Input: dimensioned drawing with shaded views. Units: mm. Origin: part minimum x, y, z. A direction names the side the tool comes from. Round coordinates to 2 decimals unless told otherwise and drop trailing zeros. Order: outer loops, then holes, each group sorted by start corner. A loop starts at its lowest first (then second) coordinate and runs counter-clockwise, first axis right, second up.
Item 1: Cut plane D-D on y = 4.05. Output: boundary loops of the cut face in (x, z) (3 decimals).
Item 2: Mould query, pull axis Y, two halves, no side actions, for the marked faces 1 and 2. Classes: released by +Y, released by -Y, zero draft, split by the parting line, or undercut.
Item 3: Cut plane B-B on y = 0.3. Output: boundary loops of the cut face in (x, z) (3 decimals), then the cut area to 3 significant figures.
Item 4: First-contact query: pin 1 (2 mm diameter, centred on y = 2.5, z = 4.5, fed in from -X) (3 decimals); pin 2 (3 mm diameter, centred on x = 4, z = 0.5, fed in from -Y) (3 decimals); pin 3 (1 mm diameter, centred on y = 4.5, z = 5.5, fed in from -X). Flat tips, straight axial feed; report the tip coordinate or a pass-through.
Item 5: Reachability of the marked faces 3 and 4 from +Z, -Z, +X, -X, +Y, -Y: full face, straight path, thin tool, end or side. Return the list, or none.
Item 6: Line query: L1, parallel to Z at x = 3.1, y = 5.25; L2, parallel to Z at x = 2.9, y = 1.5; L3, parallel to Y at x = 2.75, z = 2. Output: solid intervals per line, ascending.
Item 7: Cut plane C-C on x = 0.4. Output: boundary loops of the cut face in (y, z) (3 decimals), then the cut area to 3 significant figures.
Item 8: Cut plane A-A on z = 6.25. Output: boundary loops of the cut face in (x, y) (3 decimals), then the cut area to 3 significant figures.
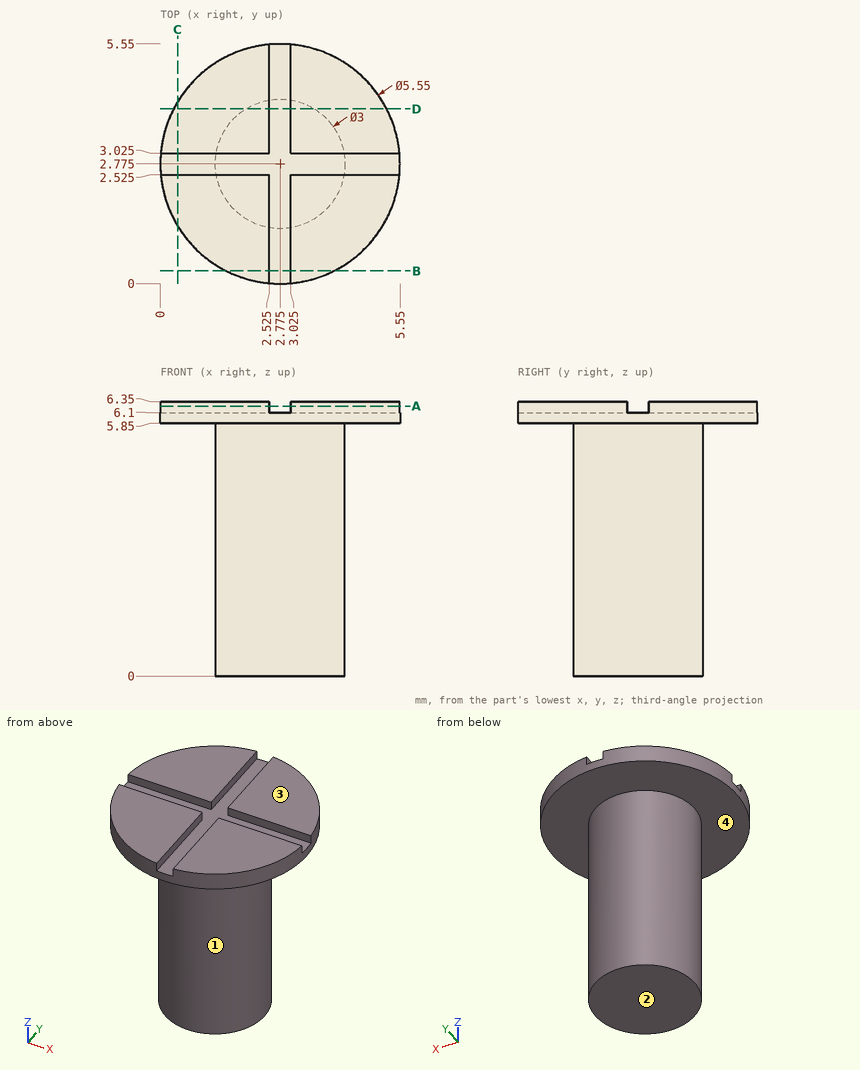
From the geometry:
1. outline: (0.31, 5.85) - (1.985, 5.85) - (1.985, 0) - (3.565, 0) - (3.565, 5.85) - (5.24, 5.85) - (5.24, 6.35) - (3.025, 6.35) - (3.025, 6.1) - (2.525, 6.1) - (2.525, 6.35) - (0.31, 6.35) - close
2. face 1: split by the parting line
2. face 2: zero draft
3. outline: (1.52, 5.85) - (4.03, 5.85) - (4.03, 6.35) - (3.025, 6.35) - (3.025, 6.1) - (2.525, 6.1) - (2.525, 6.35) - (1.52, 6.35) - close
3. area: 1.13 mm2
4. pin 1: stops at x = 1.275
4. pin 2: stops at y = 1.275
4. pin 3: stops at x = 0.36
5. face 3: +Z, +X, -X, +Y, -Y
5. face 4: -Z
6. L1: z = 5.85 to 6.35
6. L2: z = 0 to 6.1
6. L3: y = 1.28 to 4.27
7. outline: (1.34, 5.85) - (4.21, 5.85) - (4.21, 6.35) - (3.025, 6.35) - (3.025, 6.1) - (2.525, 6.1) - (2.525, 6.35) - (1.34, 6.35) - close
7. area: 1.31 mm2
8. outline: (0.011, 2.525) arc R2.775 ccw to (2.525, 0.011) - (2.525, 2.525) - close; (0.011, 3.025) - (2.525, 3.025) - (2.525, 5.539) arc R2.775 ccw to start; (3.025, 0.011) arc R2.775 ccw to (5.539, 2.525) - (3.025, 2.525) - close; (3.025, 3.025) - (5.539, 3.025) arc R2.775 ccw to (3.025, 5.539) - close
8. area: 18.9 mm2
